```python
from build123d import *

# Parameters (mm, degrees)
BOSS_EXTRUDE1_DEPTH = 80
SKETCH2_R           = 6
BOSS_EXTRUDE2_DEPTH = 30
SKETCH3_R           = 6
BOSS_EXTRUDE3_DEPTH = 30


with BuildPart() as part:
    # Sketch1 → Boss-Extrude1 (new body)
    with BuildSketch(Plane.XY):
        Polygon((3.464101615, 6), (-3.464101615, 6), (-6.92820323, 0), (-3.464101615, -6), (3.464101615, -6), (6.92820323, 0), align=None)
    extrude(amount=BOSS_EXTRUDE1_DEPTH)

    # Sketch2 → Boss-Extrude2 (add)
    with BuildSketch(Plane.XY.offset(80)):
        Circle(SKETCH2_R)
    extrude(amount=BOSS_EXTRUDE2_DEPTH)

    # Sketch3 → Boss-Extrude3 (add)
    with BuildSketch(Plane(origin=(0, 0, 0), x_dir=(-1, 0, 0), z_dir=(0, 0, -1))):
        Circle(SKETCH3_R)
    extrude(amount=BOSS_EXTRUDE3_DEPTH)


solid = part.part
```
Build history of the part. All positions in model axes, mm. A direction names the side the tool comes from. Round coordinates to 2 decimals unless told otherwise and drop trailing zeros. Loops run counter-clockwise (first coordinate to the right, second up) from the corner with the lowest first, then second, coordinate; pieces in that order, holes last. Notation, with made-up numbers: M 88.5,16.5 L 138.5,16.5 A17 cw 138.5,31.5 Z; hole C 51.25,74 d11. An arc over 180 degrees is marked long. Answer as CSV lines item,"result".
1. Wall check: probe 1 along Z at (x, y) = (4.25, 4.5); probe 2 along X at (y, z) = (0.25, -16); probe 3 along Y at (x, z) = (-3.25, 96.5). Give the ranges that are in metal, low to high. Write a range as [from, to].
Resolved:
probe 1,"z = [0, 80]"
probe 2,"x = [-5.99, 5.99]"
probe 3,"y = [-5.04, 5.04]"
2. Cut at A-A on x = 2. Write the cut outline in (y, z).
Resolved:
outline,"M -6,0 L -5.66,0 L -5.66,-30 L 5.66,-30 L 5.66,0 L 6,0 L 6,80 L 5.66,80 L 5.66,110 L -5.66,110 L -5.66,80 L -6,80 Z"
3. Cut at C-C on y = 1.75. Write the cut outline in (x, z), then the cut area to 3 significant figures.
Resolved:
outline,"M -5.92,0 L -5.74,0 L -5.74,-30 L 5.74,-30 L 5.74,0 L 5.92,0 L 5.92,80 L 5.74,80 L 5.74,110 L -5.74,110 L -5.74,80 L -5.92,80 Z"
area,"1,640 mm²"
4. 3-axis set-ups, long thin cutter, end or side, ignore diameter. For faces 1 (the flat face through (3.2, -5.4, 80)), 2 (the flat face through (-3, -5.4, 80)), 3 (the cylindrical face through (-6, 0, 95)): which of +Z, -Z, +X, -X, +Y, -Y reach the whole face in a straight line?
Resolved:
face 1,"+Z, +X, -Y"
face 2,"+Z, -X, -Y"
face 3,"+Z"
5. Cut at B-B on z = 48. Write the cut outline in (x, y), then the cut area to 3 significant figures.
Resolved:
outline,"M -6.93,0 L -3.46,-6 L 3.46,-6 L 6.93,0 L 3.46,6 L -3.46,6 Z"
area,"125 mm²"
6. Cut at D-D on z = 101.5. Write the cut outline in (x, y).
Resolved:
outline,"C 0,0 d12"
7. Flat gauge pins, fed straight in: P1, Ø5, axis at y = -2, z = 39.5, coming from the +X side; P2, Ø0.9, axis at x = -6.5, y = 1, coming from the -Z side; P3, Ø2, axis at y = 3, z = 14.5, coming from the +X side; P4, Ø6, axis at y = -3.5, z = 0, coming from the +X side. Where does each tip first touch, or does it go through?
Resolved:
P1,"stops at x = 6.93"
P2,"stops at z = 0"
P3,"stops at x = 5.77"
P4,"stops at x = 6.64"
